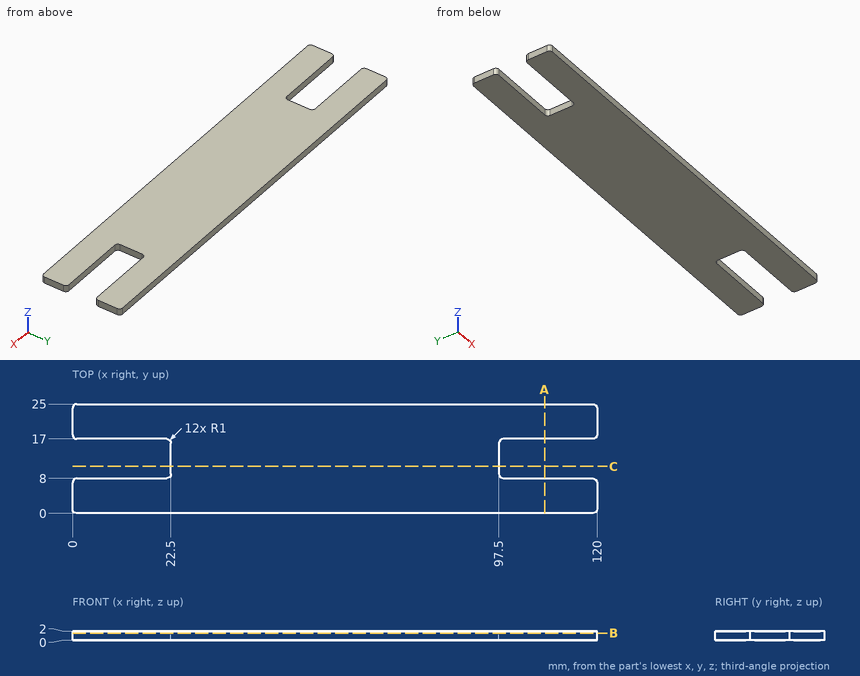
Geometry check sheet. Reference: drawing and pictorial views, mm from the part's lowest x, y, z. Coordinates: 2 decimals unless noted, no trailing zeros. Order: outer loops, then holes, each group sorted by start corner. A loop starts at its lowest first (then second) coordinate and runs counter-clockwise, first axis right, second up.
Item 1: Scan lines: line 1 along Y through (x, z) = (18.5, 1.5); line 2 along X through (y, z) = (10.25, 1.6); line 3 along Y through (x, z) = (98, 0.5). Record each from-to range of solid material in increasing order.
Item 2: Section check A-A (x = 108). Enter the section's corners in (y, z), plus the area to 3 significant figures.
Item 3: Section check C-C (y = 10.75). Enter the section's corners in (x, z).
Item 4: Depth check by flat-ended pin: pin 1 (1 mm diameter, centred on y = 11.5, z = 0.5, fed in from -X). Enter the tip coordinate at first touch or a pass-through.
Item 5: Section check B-B (z = 1.6). Enter the section's corners in (x, y), plus the area to 3 significant figures.
Check sheet entries:
1. line 1: y = 0 to 8, 17 to 25
1. line 2: x = 22.5 to 97.5
1. line 3: y = 0 to 8.13, 16.87 to 25
2. outline: (0, 0) - (8, 0) - (8, 2) - (0, 2) - close; (17, 0) - (25, 0) - (25, 2) - (17, 2) - close
2. area: 32.0 mm2
3. outline: (22.5, 0) - (97.5, 0) - (97.5, 2) - (22.5, 2) - close
4. pin 1: stops at x = 22.5
5. outline: (0, 1) arc R1 ccw to (1, 0) - (119, 0) arc R1 ccw to (120, 1) - (120, 7) arc R1 ccw to (119, 8) - (98.5, 8) arc R1 cw to (97.5, 9) - (97.5, 16) arc R1 cw to (98.5, 17) - (119, 17) arc R1 ccw to (120, 18) - (120, 24) arc R1 ccw to (119, 25) - (1, 25) arc R1 ccw to (0, 24) - (0, 18) arc R1 ccw to (1, 17) - (21.5, 17) arc R1 cw to (22.5, 16) - (22.5, 9) arc R1 cw to (21.5, 8) - (1, 8) arc R1 ccw to (0, 7) - close
5. area: 2,590 mm2
